Can you work these out from the model? Positions are in its coordinate system, mm. Round coordinates to 2 decimals unless told otherwise and drop trailing zeros. Order: outer loops, then holes, each group sorted by start corner. A loop starts at its lowest first (then second) coordinate and runs counter-clockwise, first axis right, second up. Notation, with made-up numbers: (70.25, 73.25) - (83.25, 73.25) arc R32 ccw to (83.25, 105.25) - close; hole circle Ø9 at (43, -37.75). An arc over 180 degrees is marked (long way). Write item = value, one per line.
from build123d import *

# Parameters (mm, degrees)
F0_W     = 34
F0_H     = 13.5
F1_DEPTH = 10
F2_R     = 11.5
F3_DEPTH = 10.001


with BuildPart() as f1:
    # F0 (on Front) → F1 (new body)
    with BuildSketch(Plane.XZ):
        Rectangle(F0_W, F0_H)
    extrude(amount=-F1_DEPTH)

    # F2 (on face) → F3 (cut, through all)
    with BuildSketch(Plane.XZ):
        with Locations((-0.875213, 6.75)):
            Circle(F2_R)
        Polygon((-17, -6.75), (-12.5, 6.75), (-17, 6.75), align=None)
        Polygon((11, 6.75), (17, -6.75), (17, 6.75), align=None)
    extrude(amount=-F3_DEPTH, mode=Mode.SUBTRACT)


solid = f1.part
(1) If we section it at C-C (x = 1): Write out the boundary of the cut face in (y, z).
Computed:
outline = (0, -6.75) - (10, -6.75) - (10, -4.6) - (0, -4.6) - close
(2) If I drill on line 1 (X direction, y = 4.5, z = -1.25); line 2 (X direction, y = 9.5, z = 5); line 3 (Z direction, x = 2, y = 3.5), over which ranges is the centre line in solid material (lowest first)? Write a range as from..to.
Computed:
line_1 = -15.17..-9.14, 7.39..14.56
line_2 = -13.08..-12.24, 10.49..11.78
line_3 = -6.75..-4.38
(3) Thinking about a two-plate mould opening in X: for faces 1 (the face through (14, 5, 0)), 2 (the face through (-1.128, 4.93, -4.747)), 3 (the face through (4, 0, -4)), which applies, +X half, -X half, draft (parallel to the pull), parting line (faces both ways), or undercut?
Computed:
face_1 = +X half
face_2 = undercut
face_3 = draft
(4) If we section it at D-D (z = -3.5): Write out the boundary of the cut face in (x, y).
Computed:
outline = (-15.92, 0) - (-6.09, 0) - (-6.09, 10) - (-15.92, 10) - close; (4.34, 0) - (15.56, 0) - (15.56, 10) - (4.34, 10) - close
(5) If we section it at B-B (y = 7.5): Write out the boundary of the cut face in (x, z), plus the area to 3 significant figures.
Computed:
outline = (-17, -6.75) - (17, -6.75) - (11, 6.75) - (10.62, 6.75) arc R11.5 cw to (-12.38, 6.75) - (-12.5, 6.75) - close
area = 180 mm^2
(6) Will these pins go through, and if not, where does the flat tip stop? P1, Ø6, axis at x = -10, z = -2, coming from the -Y side; P2, Ø5, axis at y = 7, z = 2.5, coming from the +X side; P3, Ø4, axis at y = 7.5, z = -3, coming from the -X side; P4, Ø1.5, axis at y = 7, z = -4, coming from the +X side.
Computed:
P1 = 0
P2 = 14
P3 = -16.42
P4 = 16.11
(7) If we section it at A-A (z = 1.25): Write out the boundary of the cut face in (x, y), plus the area to 3 significant figures.
Computed:
outline = (-14.33, 0) - (-10.97, 0) - (-10.97, 10) - (-14.33, 10) - close; (9.22, 0) - (13.44, 0) - (13.44, 10) - (9.22, 10) - close
area = 75.8 mm^2
